Here's the drawing with two shaded views (mm, measured from the low corner). I have some questions. Round coordinates to 2 decimals unless told otherwise and drop trailing zeros. Loops run counter-clockwise (first coordinate to the right, second up) from the corner with the lowest first, then second, coordinate; pieces in that order, holes last. Notation, with made-up numbers: (55, 26) -> (85, 26) arc R9 cw to (85, 33) -> close; hole circle Ø5 at (73, 70). An arc over 180 degrees is marked (long way). Use a Markdown table: item, result.
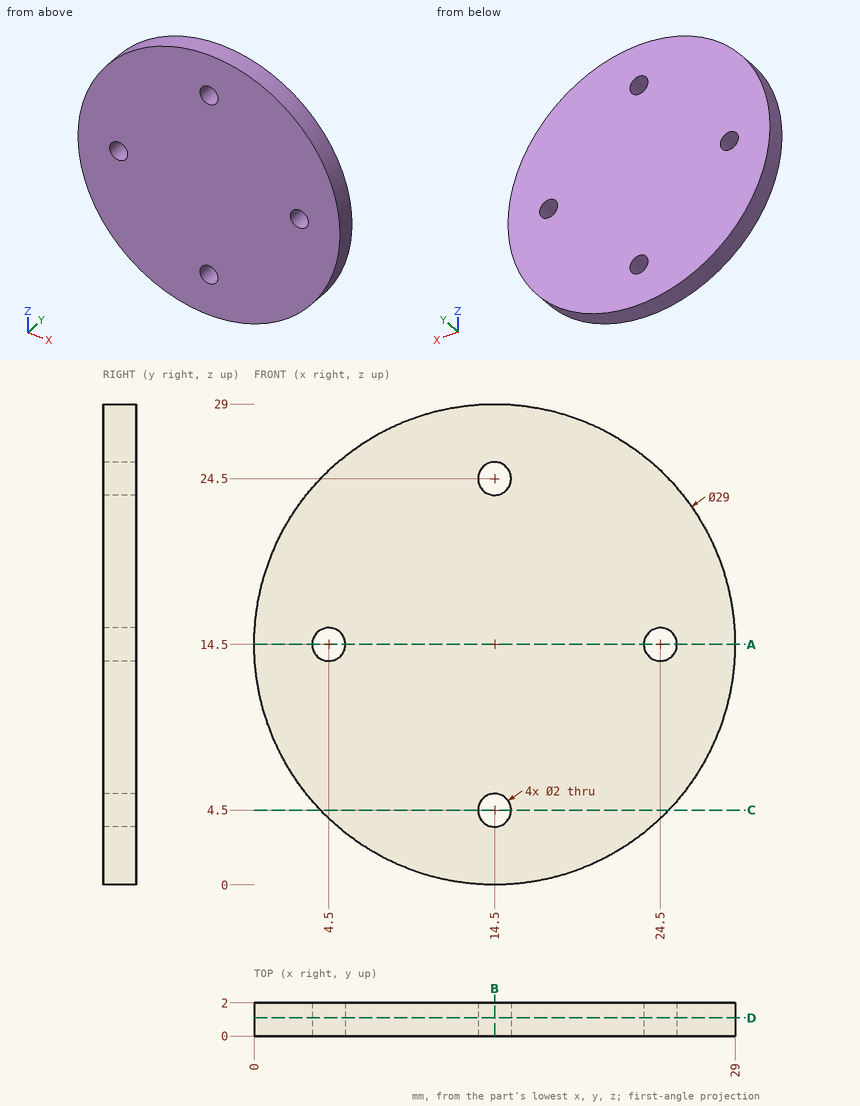
1. I want a section at D-D (y = 1.1). Please give me the cut outline in (x, z).
Answer sheet:
| item | result |
|---|---|
| outline | circle Ø29 at (14.5, 14.5); hole circle Ø2 at (4.5, 14.5); hole circle Ø2 at (14.5, 4.5); hole circle Ø2 at (14.5, 24.5); hole circle Ø2 at (24.5, 14.5) |
2. I need wall thicknesses on line 1 (X direction, y = 1, z = 14.5); line 2 (X direction, y = 1.1, z = 14); line 3 (X direction, y = 0.2, z = 23.75). Which ranges of each line are inside material? Lowest first, please.
Answer sheet:
| item | result |
|---|---|
| line 1 | x = 0 to 3.5, 5.5 to 23.5, 25.5 to 29 |
| line 2 | x = 0.01 to 3.63, 5.37 to 23.63, 25.37 to 28.99 |
| line 3 | x = 3.33 to 13.84, 15.16 to 25.67 |
3. I want a section at B-B (x = 14.5). Please give me the cut outline in (y, z), plus the area to 3 significant figures.
Answer sheet:
| item | result |
|---|---|
| outline | (0, 0) -> (2, 0) -> (2, 3.5) -> (0, 3.5) -> close; (0, 5.5) -> (2, 5.5) -> (2, 23.5) -> (0, 23.5) -> close; (0, 25.5) -> (2, 25.5) -> (2, 29) -> (0, 29) -> close |
| area | 50.0 mm² |
4. I want a section at A-A (z = 14.5). Please give me the cut outline in (x, y).
Answer sheet:
| item | result |
|---|---|
| outline | (0, 0) -> (3.5, 0) -> (3.5, 2) -> (0, 2) -> close; (5.5, 0) -> (23.5, 0) -> (23.5, 2) -> (5.5, 2) -> close; (25.5, 0) -> (29, 0) -> (29, 2) -> (25.5, 2) -> close |
5. Will this pin go through, and if not, where does the flat tip stop? pin 1 Ø1 at (y, z) = (0.5, 18) entering from +X.
Answer sheet:
| item | result |
|---|---|
| pin 1 | stops at x = 28.69 |
6. I want a section at C-C (z = 4.5). Please give me the cut outline in (x, y).
Answer sheet:
| item | result |
|---|---|
| outline | (4, 0) -> (13.5, 0) -> (13.5, 2) -> (4, 2) -> close; (15.5, 0) -> (25, 0) -> (25, 2) -> (15.5, 2) -> close |
